Autodesk Inventor part; units mm, degrees
ref_plane "YZ Plane" through (0, 0, 0) normal (1, 0, 0) x (0, 1, 0)
ref_plane "XZ Plane" through (0, 0, 0) normal (0, 1, 0) x (-1, 0, 0)
ref_plane "XY Plane" through (0, 0, 0) normal (0, 0, 1) x (1, 0, 0)
sketch "Sketch1" plane through (0, 0, 0) normal (0, 1, 0) x (-1, 0, 0)
  line L0 (0, 0) -> (25, 0)
  line L1 (25, 0) -> (25, 18.26)
  line L2 (25, 18.26) -> (0, 18.26)
  line L3 (0, 18.26) -> (0, 0)
  dimension "d0" = 25
  dimension "d1" = 18.26
extrude "Extrusion1" add sketch "Sketch1" along normal blind 8
sketch "Sketch2" plane through (0, 8, 0) normal (0, 1, 0) x (1, 0, 0)
  line L0 (0, 0) -> (-25, 0)
  line L1 (0, -18.26) -> (0, 0)
  circle A0 centre (-7, -9.13) radius 5
  dimension "d4" = 10
  dimension "d5" = 7
  dimension "d6" = 9.13
extrude "Extrusion2" cut sketch "Sketch2" against normal blind 8
sketch "Sketch3" plane through (-25, 0, 18.26) normal (0, 0, 1) x (1, 0, 0)
  line L0 (0, 0) -> (25, 0)
  line L1 (25, 0) -> (25, 8)
  circle A0 centre (4.66, 4) radius 3.5
  circle A1 centre (10.64, 4) radius 0.9905
  dimension "d9" = 7
  dimension "d10" = 1.981
  dimension "d13" = 14.36
  dimension "d14" = 20.34
  dimension "d15" = 4
extrude "Extrusion3" cut sketch "Sketch3" against normal blind 18.5
sketch "Sketch4" plane through (-25, 0, 18.26) normal (0, 0, 1) x (1, 0, 0)
  line L0 (0, 0) -> (25, 0)
  line L1 (25, 0) -> (25, 8)
  circle A0 centre (18, 4) radius 1.5
  dimension "d18" = 3
  dimension "d19" = 7
  dimension "d20" = 4
extrude "Extrusion4" cut sketch "Sketch4" against normal blind 6.5
chamfer "Chamfer1" distance 1 angle 45 2 edges at (-15.3505, 4, 18.26) (-15.3505, 4, 0)
properties part number "HeaterBlock"
Source: CAD feature listing. Evaluate the final solid. Frame: model axes, mm. A direction names the side the tool comes from. Give positions to 0.01 mm unless a question says otherwise; leave off trailing zeros. Write each loop counter-clockwise with the first axis right and the second up, starting at its lowest first coordinate (ties: lowest second). Pieces come first, ordered by that corner, then holes. Notation, with made-up numbers: (66.25, 66.5) - (117.25, 66.5) arc R16 cw to (117.25, 76.5) - close; hole circle Ø4 at (-28, -8.5). An arc over 180 degrees is marked (long way). One line per item, written item: value. Start each with the question number.
Q1. First-contact query: pin 1 Ø2.5 at (x, y) = (-14.36, 4) entering from -Z. Flat tip, straight axial feed; report the tip coordinate or a pass-through.
Q2. Draft query along X for faces 3 (the face through (-10, 4, 18.26)), 4 (the face through (-4.312, 4.056, 4.914)), 5 (the face through (-23.837, 4.154, 9.258)), 6 (the face through (-25, 4, 9)). Return one class per face: +X half, -X half, draft (parallel to the pull), parting line (faces both ways), or undercut.
Q3. Section query B-B, the plane z = 9.13. Return the cut outline in (x, y), then the cut area to 3 significant figures.
Q4. Material intervals for probe 1 along Y at (x, z) = (-7, 16.5); probe 2 along X at (y, z) = (6.75, 9.13); probe 3 along Z at (x, y) = (-7, 6.5), sorted ascending. Write a range as from..to.
Q5. Section query A-A, the plane y = 4. Return the cut outline in (x, z).
Q6. Section query D-D, the plane x = -7. Return the cut outline in (y, z).
Q7. Section query C-C, the plane x = -20.34. Return the cut outline in (y, z).
Q8. Set-up query: faces 1 (the face through (0, 4, 9)), 2 (the face through (-8.5, 4.07, 16.11)). Return all of +Z, -Z, +X, -X, +Y, -Y with unobstructed straight access to the full face (end or side cutting, diameter ignored); none if empty.
Answer:
1. pin 1: stops at z = 0.74
2. face 3: draft
2. face 4: undercut
2. face 5: undercut
2. face 6: -X half
3. outline: (-25, 0) - (-12, 0) - (-12, 8) - (-25, 8) - close; (-2, 0) - (0, 0) - (0, 8) - (-2, 8) - close; hole circle Ø7 at (-20.34, 4); hole circle Ø1.98 at (-14.36, 4)
3. area: 78.4 mm2
4. probe 1: y = 0..2.5, 5.5..8
4. probe 2: x = -25..-22.51, -18.17..-12, -2..0
4. probe 3: z = 0..4.13, 14.13..18.26
5. outline: (-25, 0) - (-23.84, 0) - (-23.84, 18.26) - (-25, 18.26) - close; (-16.84, 0) - (-16.35, 0) - (-15.35, 1) - (-15.35, 17.26) - (-16.35, 18.26) - (-16.84, 18.26) - close; (-13.37, 1) - (-12.37, 0) - (0, 0) - (0, 18.26) - (-5.5, 18.26) - (-5.5, 13.9) arc R5 cw (long way) to (-8.5, 13.9) - (-8.5, 18.26) - (-12.37, 18.26) - (-13.37, 17.26) - close
6. outline: (0, 0) - (8, 0) - (8, 4.13) - (0, 4.13) - close; (0, 14.13) - (2.5, 14.13) - (2.5, 18.26) - (0, 18.26) - close; (5.5, 14.13) - (8, 14.13) - (8, 18.26) - (5.5, 18.26) - close
7. outline: (0, 0) - (0.5, 0) - (0.5, 18.26) - (0, 18.26) - close; (7.5, 0) - (8, 0) - (8, 18.26) - (7.5, 18.26) - close
8. face 1: +Z, -Z, +X, +Y, -Y
8. face 2: +Z
